from build123d import *

# Parameters (mm, degrees)
F0_R     = 2.54
F1_DEPTH = 3.175
F2_SIZE2 = 2.54
F2_SIZE  = 2.54
F3_R     = 1.905


with BuildPart() as f1:
    # F0 (on Top) → F1 (new body)
    with BuildSketch(Plane.XY):
        with BuildLine():
            ThreePointArc((5.5358016583, -11.43), (10.7609172718, -6.7448246434), (12.7, 0))
            ThreePointArc((12.7, 0), (-6.7448246434, 10.7609172718), (-5.5358016583, -11.43))
            Line((-5.5358016583, -11.43), (5.5358016583, -11.43))
        make_face()
        Circle(F0_R, mode=Mode.SUBTRACT)
    extrude(amount=F1_DEPTH)

    # F2
    f2_edges = [f1.edges().sort_by_distance(p)[0] for p in [
        (-2.54, 0, 3.175),
    ]]
    chamfer(f2_edges, length=F2_SIZE, length2=F2_SIZE2)

    # F3
    f3_edges = [f1.edges().sort_by_distance(p)[0] for p in [
        (-5.535802, -11.43, 1.5875),
        (5.535802, -11.43, 1.5875),
    ]]
    fillet(f3_edges, radius=F3_R)


solid = f1.part
Geometry check sheet. Reference: the model listing, model coordinates, mm. Give positions to 0.01 mm unless a question says otherwise; leave off trailing zeros. Loops run counter-clockwise (first coordinate to the right, second up) from the corner with the lowest first, then second, coordinate; pieces in that order, holes last. Notation, with made-up numbers: (16, -35) -> (59, -35) arc R30 ccw to (59, -4) -> close; hole circle Ø5 at (66, 58.5). An arc over 180 degrees is marked (long way). Answer in a Markdown table with one row per item. Add a question column.
1) Draft check along X on faces 1 (the face through (3, 1, 0)), 2 (the face through (1.25, -2.39, 0.79)), 3 (the face through (-5.536, -11.375, 1.61)), 4 (the face through (5.55, -11.37, 1.61)). Enter one of: pulls with the +X half, pulls with the -X half, needs draft (parallel to the pull), parting line crosses it, or undercut.
2) Gauge pin test, flat ends, axial feed: P1, Ø1.5, axis at x = -7.5, z = 1, coming from the -Y side; P2, Ø1.5, axis at y = 2.5, z = 1.5, coming from the +X side. Record the tip position at first contact, or that the pin passes through.
3) Cross-section at D-D on x = 10. Record the boundary of the cut face in (y, z) (3 decimals).
4) Material ranges on probe 1 along Y at (x, z) = (0, 0.45); probe 2 along X at (y, z) = (1.75, 0.95); probe 3 along Y at (x, z) = (4, 3), recorded low to high. Write a range as from..to.
5) Cross-section at B-B on z = 1.4. Record the boundary of the cut face in (x, y) (3 decimals), and give its area (3 significant figures).
6) Cross-section at C-C on y = 5.75. Record the boundary of the cut face in (x, z) (3 decimals), and give its area (3 significant figures).
7) Cross-section at A-A on x = 0. Record the boundary of the cut face in (y, z) (3 decimals), and give its area (3 significant figures).
Outcome:
| question | item | result |
|---|---|---|
| 1 | face 1 | needs draft |
| 1 | face 2 | undercut |
| 1 | face 3 | pulls with the -X half |
| 1 | face 4 | pulls with the +X half |
| 2 | P1 | stops at y = -10.76 |
| 2 | P2 | stops at x = 12.58 |
| 3 | outline | (-7.829, 0) -> (7.829, 0) -> (7.829, 3.175) -> (-7.829, 3.175) -> close |
| 4 | probe 1 | y = -11.43..-2.54, 2.54..12.7 |
| 4 | probe 2 | x = -12.58..-2.26, 2.26..12.58 |
| 4 | probe 3 | y = -11.43..-2.84, 2.84..12.05 |
| 5 | outline | (-5.976, -11.206) arc R1.905 ccw to (-5.08, -11.43) -> (5.08, -11.43) arc R1.905 ccw to (5.976, -11.206) arc R12.7 ccw (long way) to start; hole circle Ø6.61 at (0, 0) |
| 5 | area | 463 mm^2 |
| 6 | outline | (-11.324, 0) -> (11.324, 0) -> (11.324, 3.175) -> (-11.324, 3.175) -> close |
| 6 | area | 71.9 mm^2 |
| 7 | outline | (-11.43, 0) -> (-2.54, 0) -> (-2.54, 0.635) -> (-5.08, 3.175) -> (-11.43, 3.175) -> close; (2.54, 0) -> (12.7, 0) -> (12.7, 3.175) -> (5.08, 3.175) -> (2.54, 0.635) -> close |
| 7 | area | 54.0 mm^2 |
